```python
from build123d import *

# Parameters (mm, degrees)
SKETCH1_R           = 127
BOSS_EXTRUDE1_DEPTH = 5


with BuildPart() as part:
    # Sketch1 → Boss-Extrude1 (new body)
    with BuildSketch(Plane.XY):
        with BuildLine():
            Line((-2045.288455612, -640.670506336), (-1137.971443758, -640.670506336))
            ThreePointArc((-1137.971443758, -640.670506336), (-3061.28152044, -1101.624467207), (-1134.61767518, -1548.353280331))
            Line((-1134.61767518, -1548.353280331), (-2045.288455612, -1555.070506336))
            ThreePointArc((-2045.288455612, -1555.070506336), (-2502.488455612, -1097.870506336), (-2045.288455612, -640.670506336))
        make_face()
        with Locations((-2045.288455612, -386.670506336)):
            Circle(SKETCH1_R, mode=Mode.SUBTRACT)
        with Locations((-2756.488455612, -1097.870506336)):
            Circle(SKETCH1_R, mode=Mode.SUBTRACT)
        with Locations(Location((-2045.288455612, -1809.070506336, 0), (0, 0, 180))):
            Circle(SKETCH1_R, mode=Mode.SUBTRACT)
    extrude(amount=BOSS_EXTRUDE1_DEPTH)


solid = part.part
```
Build history of the part. All positions in model axes, mm. Round coordinates to 2 decimals unless told otherwise and drop trailing zeros. Loops run counter-clockwise (first coordinate to the right, second up) from the corner with the lowest first, then second, coordinate; pieces in that order, holes last.
Item 1: Saw through at A-A (y = -1128.5). List the corners of the cut face in (x, z), then the cut area to 3 significant figures.
Item 2: Pin check, flat tips, straight feed: P1, Ø1, axis at x = -1785, z = 3, coming from the +Y side; P2, Ø1.5, axis at x = -1542, z = 2, coming from the -Y side; P3, Ø2, axis at y = -498, z = 0.5, coming from the -X side. Stop position of each tip, or through.
Item 3: Saw through at C-C (x = -1348.5). List the corners of the cut face in (y, z), then the cut area to 3 significant figures.
Item 4: Two-plate mould, pull along X, no slides. Class faces 1 (the face through (-3060.708, -1063.532, 2.465)), 2 (the face through (-2166.424, -1847.218, 2.465)), 3 (the face through (-2540, -1084, 0)): released by +X, released by -X, zero draft, split by the parting line, or undercut.
Item 5: Saw through at B-B (x = -2127.5). List the corners of the cut face in (y, z).
Item 6: Saw through at D-D (z = 2.2). List the corners of the cut face in (x, y), then the cut area to 3 significant figures.
Item 7: Drill centre lines: line 1 along X through (y, z) = (-408.5, 1.1); line 2 along X through (y, z) = (-1866.5, 2.55); line 3 along Y through (x, z) = (-2143.5, 1.4). Where is each one in solid material? Low to high.
Worked answers:
1. outline: (-3060.83, 0) - (-2879.74, 0) - (-2879.74, 5) - (-3060.83, 5) - close; (-2633.24, 0) - (-2501.46, 0) - (-2501.46, 5) - (-2633.24, 5) - close
1. area: 1,560 mm2
2. P1: stops at y = -115.65
2. P2: stops at y = -1980.88
2. P3: stops at x = -2866.03
3. outline: (-1837.29, 0) - (-1549.93, 0) - (-1549.93, 5) - (-1837.29, 5) - close; (-640.67, 0) - (-358.45, 0) - (-358.45, 5) - (-640.67, 5) - close
3. area: 2,850 mm2
4. face 1: split by the parting line
4. face 2: undercut
4. face 3: zero draft
5. outline: (-2110.54, 0) - (-1905.87, 0) - (-1905.87, 5) - (-2110.54, 5) - close; (-1712.27, 0) - (-1547.62, 0) - (-1547.62, 5) - (-1712.27, 5) - close; (-648.12, 0) - (-483.47, 0) - (-483.47, 5) - (-648.12, 5) - close; (-289.87, 0) - (-85.2, 0) - (-85.2, 5) - (-289.87, 5) - close
6. outline: (-2045.29, -1555.07) arc R457.2 cw to (-2045.29, -640.67) - (-1137.97, -640.67) arc R1016 ccw (long way) to (-1134.62, -1548.35) - close; hole circle Ø254 at (-2756.49, -1097.87); hole circle Ø254 at (-2045.29, -1809.07); hole circle Ø254 at (-2045.29, -386.67)
6. area: 1,870,000 mm2
7. line 1: x = -2791.63 to -2170.4, -1920.18 to -1298.95
7. line 2: x = -2709.72 to -2158.56, -1932.02 to -1380.86
7. line 3: y = -2109.11 to -1889.59, -1728.55 to -1544.4, -651.34 to -467.19, -306.15 to -86.63
